Geometry check sheet. Reference: the model listing, model coordinates, mm. Give positions to 0.01 mm unless a question says otherwise; leave off trailing zeros. Order: outer loops, then holes, each group sorted by start corner. A loop starts at its lowest first (then second) coordinate and runs counter-clockwise, first axis right, second up. Notation, with made-up numbers: M 10,30.25 L 17,30.25 A23 ccw 17,66.25 Z; hole C 7,22 d11. An arc over 180 degrees is marked long. Answer as a JSON object with one key per item and string values. Group by question number.
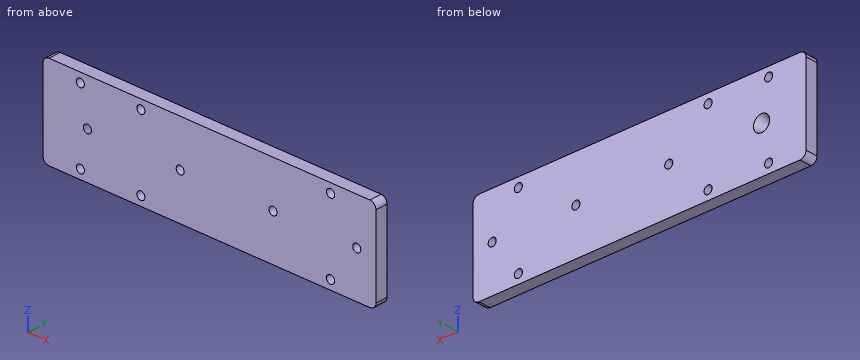
from build123d import *

# Parameters (mm, degrees)
SKETCH1_R           = 2
BOSS_EXTRUDE1_DEPTH = 3


with BuildPart() as part:
    # Sketch1 → Boss-Extrude1 (new, symmetric)
    with BuildSketch(Plane(origin=(0, 0, 0), x_dir=(1, 0, 0), z_dir=(0, 1, 0))):
        with BuildLine():
            Line((-79.5, 22.5), (79.5, 22.5))
            ThreePointArc((79.5, 22.5), (81.621320344, 21.621320344), (82.5, 19.5))
            Line((82.5, 19.5), (82.5, -19.5))
            ThreePointArc((82.5, -19.5), (81.621320344, -21.621320344), (79.5, -22.5))
            Line((79.5, -22.5), (-79.5, -22.5))
            ThreePointArc((-79.5, -22.5), (-81.621320344, -21.621320344), (-82.5, -19.5))
            Line((-82.5, -19.5), (-82.5, 19.5))
            ThreePointArc((-82.5, 19.5), (-81.621320344, 21.621320344), (-79.5, 22.5))
        make_face()
        with Locations(Location((-64, 18, 0), (0, 0, 270))):
            Circle(SKETCH1_R, mode=Mode.SUBTRACT)
        with Locations(Location((-34, 18, 0), (0, 0, 270))):
            Circle(SKETCH1_R, mode=Mode.SUBTRACT)
        with Locations(Location((60, 18, 0), (0, 0, 270))):
            Circle(SKETCH1_R, mode=Mode.SUBTRACT)
        with Locations(Location((-60.5, 0, 0), (0, 0, 270))):
            Circle(SKETCH1_R, mode=Mode.SUBTRACT)
        with Locations(Location((-14.5, 0, 0), (0, 0, 270))):
            Circle(SKETCH1_R, mode=Mode.SUBTRACT)
        with Locations(Location((31.5, 0, 0), (0, 0, 270))):
            Circle(SKETCH1_R, mode=Mode.SUBTRACT)
        with Locations(Location((73, 0, 0), (0, 0, 270))):
            Circle(SKETCH1_R, mode=Mode.SUBTRACT)
        with Locations(Location((60, -18, 0), (0, 0, 270))):
            Circle(SKETCH1_R, mode=Mode.SUBTRACT)
        with Locations(Location((-34, -18, 0), (0, 0, 270))):
            Circle(SKETCH1_R, mode=Mode.SUBTRACT)
        with Locations(Location((-64, -18, 0), (0, 0, 270))):
            Circle(SKETCH1_R, mode=Mode.SUBTRACT)
    extrude(amount=BOSS_EXTRUDE1_DEPTH, both=True)

    # Sketch7 → Cut-Revolve1 (revolve, cut)
    with BuildSketch(Plane.XY, mode=Mode.PRIVATE) as cut_revolve1_sk:
        Polygon((-58.5, -3), (-56.5, 3), (-58.5, 3), align=None)
    revolve(cut_revolve1_sk.sketch.rotate(Axis((-60.5, 0, 0), (0, -1, 0)), 180), axis=Axis((-60.5, 0, 0), (0, -1, 0)), mode=Mode.SUBTRACT)


solid = part.part
1. Cross-section at B-B (x = 73). Record the cut outline in (y, z), and give its area (3 significant figures).
2. Cross-section at A-A (z = 18). Record the cut outline in (x, y).
3. Cross-section at D-D (z = 0). Record the cut outline in (x, y), and give its area (3 significant figures).
4. Thickness scan on line 1 along X through (y, z) = (-0.6, -18); line 2 along Z through (x, y) = (-32.5, 1.25); line 3 along X through (y, z) = (-0.25, -1). Record the ranges inside material, lowest first. Write a range as [from, to].
5. Cross-section at C-C (y = -1.5). State how many separate pieces and enclosed holes the cut face has, and give its area (3 significant figures).
Report:
{
 "1": {"outline": "M -3,-22.5 L 3,-22.5 L 3,-2 L -3,-2 Z; M -3,2 L 3,2 L 3,22.5 L -3,22.5 Z", "area": "246 mm2"},
 "2": {"outline": "M -82.5,-3 L -66,-3 L -66,3 L -82.5,3 Z; M -62,-3 L -36,-3 L -36,3 L -62,3 Z; M -32,-3 L 58,-3 L 58,3 L -32,3 Z; M 62,-3 L 82.5,-3 L 82.5,3 L 62,3 Z"},
 "3": {"outline": "M -82.5,-3 L -62.5,-3 L -64.5,3 L -82.5,3 Z; M -58.5,-3 L -16.5,-3 L -16.5,3 L -56.5,3 Z; M -12.5,-3 L 29.5,-3 L 29.5,3 L -12.5,3 Z; M 33.5,-3 L 71,-3 L 71,3 L 33.5,3 Z; M 75,-3 L 82.5,-3 L 82.5,3 L 75,3 Z", "area": "882 mm2"},
 "4": {"line 1": "x = [-82.5, -66], [-62, -36], [-32, 58], [62, 82.5]", "line 2": "z = [-22.5, -19.32], [-16.68, 16.68], [19.32, 22.5]", "line 3": "x = [-82.5, -63.24], [-57.76, -16.23], [-12.77, 29.77], [33.23, 71.27], [74.73, 82.5]"},
 "5": {"separate pieces": "1", "enclosed holes": "10", "area": "7,280 mm2"}
}
